```python
from build123d import *

# Parameters (mm, degrees)
BOSS_EXTRUDE1_DEPTH = 8


with BuildPart() as part:
    # Sketch2 → Boss-Extrude1 (new body)
    with BuildSketch(Plane(origin=(0, 0, 0), x_dir=(1, 0, 0), z_dir=(0, 1, 0))):
        with BuildLine():
            ThreePointArc((26, 0), (30, 4), (34, 0))
            Line((34, 0), (37.5, 0))
            Line((37.5, 0), (37.5, 7.5))
            Line((37.5, 7.5), (-37.5, 7.5))
            Line((-37.5, 7.5), (-37.5, 0))
            Line((-37.5, 0), (-34, 0))
            ThreePointArc((-34, 0), (-30, 4), (-26, 0))
            Line((-26, 0), (26, 0))
        make_face()
        with BuildLine():
            Line((37.5, 0), (34, 0))
            ThreePointArc((34, 0), (30, -4), (26, 0))
            Line((26, 0), (-26, 0))
            ThreePointArc((-26, 0), (-30, -4), (-34, 0))
            Line((-34, 0), (-37.5, 0))
            Line((-37.5, 0), (-37.5, -7.5))
            Line((-37.5, -7.5), (37.5, -7.5))
            Line((37.5, -7.5), (37.5, 0))
        make_face()
    extrude(amount=BOSS_EXTRUDE1_DEPTH)


solid = part.part
```
CAD build for the part. Positions are in the model's coordinates, mm. Round coordinates to 2 decimals unless told otherwise and drop trailing zeros. Order: outer loops, then holes, each group sorted by start corner. A loop starts at its lowest first (then second) coordinate and runs counter-clockwise, first axis right, second up.
Item 1: Saw through at A-A on z = 0. Write the cut outline in (x, y).
Item 2: Saw through at D-D on x = 31.5. Write the cut outline in (y, z), then the cut area to 3 significant figures.
Item 3: Saw through at C-C on y = 1.5. Write the cut outline in (x, z).
Item 4: Mould opens along X. For faces 1 (the face through (-1, 8, 0)), 2 (the face through (37.5, 4, 0)), 3 (the face through (26.8, 3.9, -2.4)) say: pulls with the +X half, pulls with the -X half, needs draft (parallel to the pull), parting line crosses it, or undercut.
Item 5: Saw through at B-B on x = -30. Write the cut outline in (y, z).
Item 6: Probe line 1 along Z through (x, y) = (-30, 2.5); line 2 along X through (y, z) = (6, 1.75); line 3 along X through (y, z) = (4.75, 2). List the from-to ranges inside material, lowest first.
Reported:
1. outline: (-37.5, 0) - (-34, 0) - (-34, 8) - (-37.5, 8) - close; (-26, 0) - (26, 0) - (26, 8) - (-26, 8) - close; (34, 0) - (37.5, 0) - (37.5, 8) - (34, 8) - close
2. outline: (0, -7.5) - (8, -7.5) - (8, -3.71) - (0, -3.71) - close; (0, 3.71) - (8, 3.71) - (8, 7.5) - (0, 7.5) - close
2. area: 60.7 mm2
3. outline: (-37.5, -7.5) - (37.5, -7.5) - (37.5, 7.5) - (-37.5, 7.5) - close; hole circle Ø8 at (-30, 0); hole circle Ø8 at (30, 0)
4. face 1: needs draft
4. face 2: pulls with the +X half
4. face 3: undercut
5. outline: (0, -7.5) - (8, -7.5) - (8, -4) - (0, -4) - close; (0, 4) - (8, 4) - (8, 7.5) - (0, 7.5) - close
6. line 1: z = -7.5 to -4, 4 to 7.5
6. line 2: x = -37.5 to -33.6, -26.4 to 26.4, 33.6 to 37.5
6. line 3: x = -37.5 to -33.46, -26.54 to 26.54, 33.46 to 37.5
